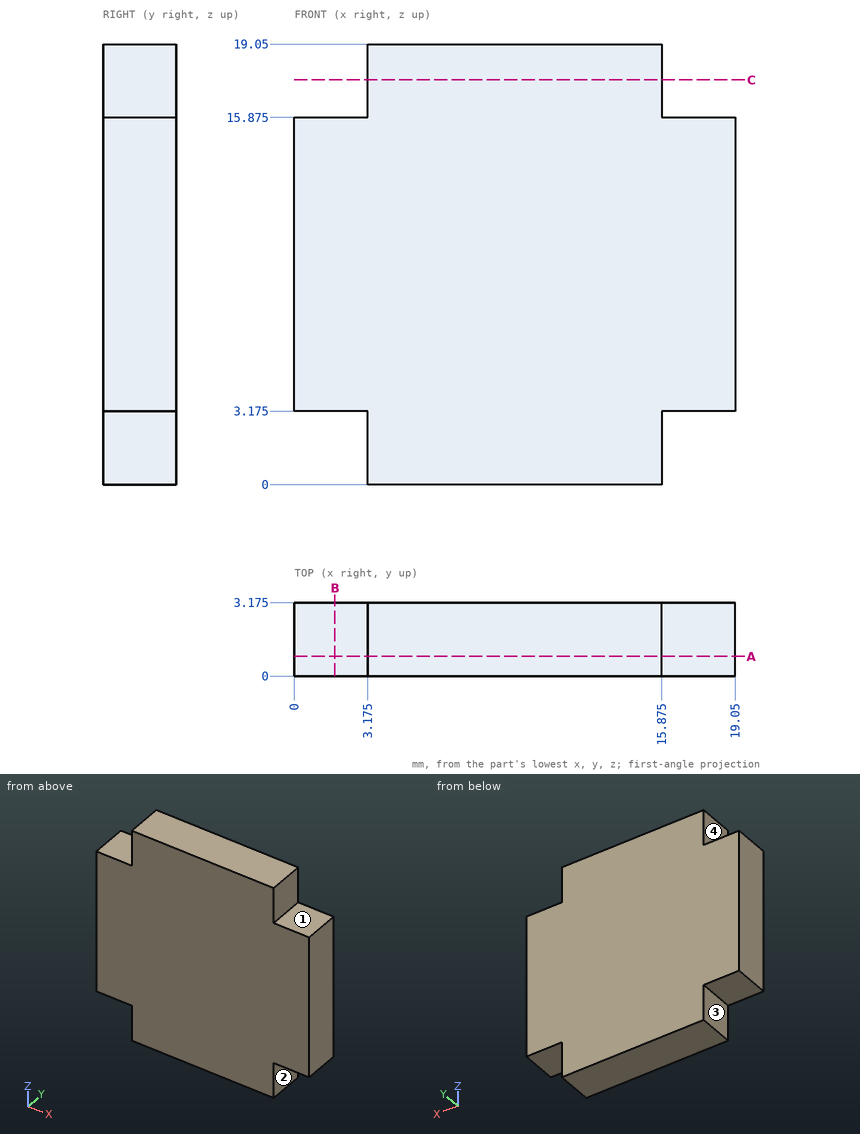
Here's the drawing with two shaded views (mm, measured from the low corner). I have some questions. A direction names the side the tool comes from. Coordinates: 2 decimals unless noted, no trailing zeros. Order: outer loops, then holes, each group sorted by start corner. A loop starts at its lowest first (then second) coordinate and runs counter-clockwise, first axis right, second up.
Item 1: I need wall thicknesses on probe 1 along X at (y, z) = (0.9, 16) (3 decimals). Which ranges of the line are inside material? Lowest first, please.
Response values:
probe 1: x = 3.175 to 15.875
Item 2: Which directions (+Z, -Z, +X, -X, +Y, -Y) give clear straight access to the entire face, cutting with the end or side of a thin tool? Please do the marked faces 1, 2, 3 and 4.
Response values:
face 1: +Z, +X, +Y, -Y
face 2: -Z, +X, +Y, -Y
face 3: -Z, -X, +Y, -Y
face 4: +Z, -X, +Y, -Y
Item 3: If we section it at B-B, the plane x = 1.75: List the corners of the cut face in (y, z) for me (3 decimals).
Response values:
outline: (0, 3.175) - (3.175, 3.175) - (3.175, 15.875) - (0, 15.875) - close
Item 4: If we section it at A-A, the plane y = 0.85: List the corners of the cut face in (x, z) for me (3 decimals), then the cut area to 3 significant figures.
Response values:
outline: (0, 3.175) - (3.175, 3.175) - (3.175, 0) - (15.875, 0) - (15.875, 3.175) - (19.05, 3.175) - (19.05, 15.875) - (15.875, 15.875) - (15.875, 19.05) - (3.175, 19.05) - (3.175, 15.875) - (0, 15.875) - close
area: 323 mm2
Item 5: I'm going to push flat-ended pins straight in: pin 1 Ø1 at (y, z) = (2, 2) entering from +X (3 decimals); pin 2 Ø1.6 at (y, z) = (1.5, 1) entering from -X (3 decimals); pin 3 Ø1.5 at (x, z) = (15.5, 12.5) entering from -Y; pin 4 Ø1 at (x, y) = (17, 0.5) entering from +Z (3 decimals). Where does each tip first touch, or does it pass through?
Response values:
pin 1: stops at x = 15.875
pin 2: stops at x = 3.175
pin 3: stops at y = 0
pin 4: stops at z = 15.875
Item 6: If we section it at C-C, the plane z = 17.5: List the corners of the cut face in (x, y) for me (3 decimals).
Response values:
outline: (3.175, 0) - (15.875, 0) - (15.875, 3.175) - (3.175, 3.175) - close
